Part model, mm, in its own coordinate system. A direction names the side the tool comes from. Give positions to 0.01 mm unless a question says otherwise; leave off trailing zeros. Order: outer loops, then holes, each group sorted by start corner. A loop starts at its lowest first (then second) coordinate and runs counter-clockwise, first axis right, second up. Notation, with made-up numbers: M -21,7.5 L 0,7.5 A18 cw 0,42.5 Z; hole C -13,28 d9. An arc over 180 degrees is marked long. Write each question's results on one line, items separated by ' | '. Start each with the question number.
from build123d import *

# Parameters (mm, degrees)
SKETCH_1_W                   = 54
SKETCH_1_H                   = 20
EXTRUDE_1_DEPTH              = 12
HOLE_WIZARD_M6_1_D           = 5
HOLE_WIZARD_M5_1_D           = 5.8
HOLE_WIZARD_M5_1_CBORE_D     = 10
HOLE_WIZARD_M5_1_CBORE_DEPTH = 5


with BuildPart() as part:
    # 草图1 → 凸台-拉伸1 (new body)
    with BuildSketch(Plane.XY):
        with Locations((27, 10)):
            Rectangle(SKETCH_1_W, SKETCH_1_H)
    extrude(amount=EXTRUDE_1_DEPTH)

    # M6 螺纹孔1 (through all)
    with Locations(Plane.XY.offset(12)):
        with Locations((27, 12)):
            Hole(HOLE_WIZARD_M6_1_D / 2)

    # M5 六角凹头螺钉的柱形沉头孔1 (through all)
    with Locations(Plane(origin=(0, 20, 0), x_dir=(-1, 0, 0), z_dir=(0, 1, 0))):
        with Locations((-47, 6), (-7, 6)):
            CounterBoreHole(HOLE_WIZARD_M5_1_D / 2, HOLE_WIZARD_M5_1_CBORE_D / 2, HOLE_WIZARD_M5_1_CBORE_DEPTH)


solid = part.part
(1) Tool access for faces 1 (the flat face through (44.8, 15, 3.8)), 2 (the flat face through (54, 10, 6)): list every direction of +Z, -Z, +X, -X, +Y, -Y with a clear straight run to the whole face (end or side of a thin tool).
(2) Pull direction X, two halves, no side cores. Call faces 3 (the cylindrical face through (52, 18, 6)), 4 (the flat face through (0, 10, 6)), 5 (the flat face through (27, 20, 6)): +X half, -X half, draft (parallel to the pull), parting line (faces both ways), or undercut.
(3) Saw through at A-A on z = 6. Give the cut face in (x, y).
(4) Saw through at C-C on x = 47. Give the cut face in (y, z).
(5) Probe L1, parallel to Y at x = 27, z = 9; L2, parallel to X at y = 9.25, z = 7.5; L3, parallel to Z at x = 47, y = 4.5. List the from-to ranges inside material, lowest first.
(6) Saw through at D-D on x = 27. Give the cut face in (y, z).
(7) Drop flat-ended pins along their axis: P1, Ø3, axis at x = 47.5, z = 4, coming from the +Y side; P2, Ø4, axis at x = 27, y = 12, coming from the -Z side (3 decimals). Give the stop position or say it passes through.
(8) Saw through at B-B on y = 12. Give the cut face in (x, z), plus the area to 3 significant figures.
Taken from the geometry:
1) face 1: +Y | face 2: +Z, -Z, +X, +Y, -Y
2) face 3: undercut | face 4: -X half | face 5: draft
3) outline: M 0,0 L 4.1,0 L 4.1,15 L 2,15 L 2,20 L 0,20 Z; M 9.9,0 L 44.1,0 L 44.1,15 L 42,15 L 42,20 L 12,20 L 12,15 L 9.9,15 Z; M 49.9,0 L 54,0 L 54,20 L 52,20 L 52,15 L 49.9,15 Z; hole C 27,12 d5
4) outline: M 0,0 L 20,0 L 20,1 L 15,1 L 15,3.1 L 0,3.1 Z; M 0,8.9 L 15,8.9 L 15,11 L 20,11 L 20,12 L 0,12 Z
5) L1: y = 0 to 9.5, 14.5 to 20 | L2: x = 0 to 4.52, 9.48 to 44.52, 49.48 to 54 | L3: z = 0 to 3.1, 8.9 to 12
6) outline: M 0,0 L 9.5,0 L 9.5,12 L 0,12 Z; M 14.5,0 L 20,0 L 20,12 L 14.5,12 Z
7) P1: stops at y = 15 | P2: passes through
8) outline: M 0,0 L 24.5,0 L 24.5,12 L 0,12 Z; M 29.5,0 L 54,0 L 54,12 L 29.5,12 Z; hole C 7,6 d5.8; hole C 47,6 d5.8 | area: 535 mm²
